Check sheet for the modelled part. Datum: model origin and axes. Units: mm. A direction names the side the tool comes from. Round coordinates to 2 decimals unless told otherwise and drop trailing zeros. Write each loop counter-clockwise with the first axis right and the second up, starting at its lowest first coordinate (ties: lowest second). Pieces come first, ordered by that corner, then holes. Notation, with made-up numbers: (2.25, 68.5) - (54.25, 68.5) arc R26 ccw to (54.25, 107.5) - close; hole circle Ø3 at (74.5, 83.5). An arc over 180 degrees is marked (long way). Use one line per item in the form item = value. Start each with the question number.
1) Section check C-C (x = 61.5). Record the boundary of the cut face in (y, z), then the cut area to 3 significant figures.
2) Section check A-A (z = 30). Record the boundary of the cut face in (x, y), then the cut area to 3 significant figures.
3) Scan lines: probe 1 along Z at (x, y) = (30, -17.5); probe 2 along Y at (x, z) = (30, 14); probe 3 along X at (y, z) = (9.5, 22). Record each from-to range of solid material in increasing order.
4) Section check B-B (x = 30). Record the boundary of the cut face in (y, z).
5) Draft check along X on faces 1 (the face through (28.37, 19.93, 22.68)), 2 (the face through (60, -20, 30)), 3 (the face through (40, -15, 30)). Enter one of: +X half, -X half, draft (parallel to the pull), parting line (faces both ways), or undercut.
6) Gauge pin test, flat ends, axial feed: P1, Ø24, axis at x = 30, z = 30, coming from the +Y side; P2, Ø12, axis at y = 9.5, z = 36.5, coming from the +X side; P3, Ø1, axis at y = -4.5, z = 31.5, coming from the +X side; P4, Ø12, axis at x = 63.5, y = 1.5, coming from the +Z side. Record the tip position at first contact, or that the pin passes through.
7) Section check D-D (y = 10). Record the boundary of the cut face in (x, z).
8) Set-up check for faces 4 (the face through (10, 0, 30)), 5 (the face through (60, 20, 30)): record each of +Z, -Z, +X, -X, +Y, -Y from which the full face is reachable in a straight line by a thin tool's end or side.
from build123d import *

# Parameters (mm, degrees)
F1_DEPTH = 25
F2_W     = 20
F2_H     = 30
F2_W_2   = 40
F3_DEPTH = 40
F4_R     = 7.5
F5_DEPTH = 50.001


with BuildPart() as f1:
    # F0 (on Front) → F1 (new body, symmetric)
    with BuildSketch(Plane.XZ):
        Polygon((0, 50), (0, 0), (100, 0), (100, 10), (70, 10), (50, 50), align=None)
    extrude(amount=F1_DEPTH, both=True)

    # F2 (on face) → F3 (cut, through all)
    with BuildSketch(Plane.XY.offset(50)):
        with Locations((60, 0)):
            Rectangle(F2_W, F2_H)
        with Locations((30, 0)):
            Rectangle(F2_W_2, F2_H)
    extrude(amount=-F3_DEPTH, mode=Mode.SUBTRACT)

    # F4 (on face) → F5 (cut, through all)
    with BuildSketch(Plane.XZ.offset(25)):
        with Locations((30, 30)):
            Circle(F4_R)
    extrude(amount=-F5_DEPTH, mode=Mode.SUBTRACT)


solid = f1.part
Results are:
q1.outline = (-25, 0) - (25, 0) - (25, 27) - (15, 27) - (15, 10) - (-15, 10) - (-15, 27) - (-25, 27) - close
q1.area = 840 mm²
q2.outline = (0, -25) - (22.5, -25) - (22.5, -15) - (10, -15) - (10, 15) - (22.5, 15) - (22.5, 25) - (0, 25) - close; (37.5, -25) - (60, -25) - (60, -15) - (37.5, -15) - close; (37.5, 15) - (60, 15) - (60, 25) - (37.5, 25) - close
q2.area = 1,200 mm²
q3.probe_1 = 0 to 22.5, 37.5 to 50
q3.probe_2 = -25 to -15, 15 to 25
q3.probe_3 = 0 to 10
q4.outline = (-25, 0) - (25, 0) - (25, 22.5) - (15, 22.5) - (15, 10) - (-15, 10) - (-15, 22.5) - (-25, 22.5) - close; (-25, 37.5) - (-15, 37.5) - (-15, 50) - (-25, 50) - close; (15, 37.5) - (25, 37.5) - (25, 50) - (15, 50) - close
q5.face_1 = undercut
q5.face_2 = +X half
q5.face_3 = draft
q6.P1 = 25
q6.P2 = 57.95
q6.P3 = 10
q6.P4 = 10
q7.outline = (0, 0) - (100, 0) - (100, 10) - (10, 10) - (10, 50) - (0, 50) - close
q8.face_4 = +Z, +X
q8.face_5 = +Z, +X, +Y, -Y
